Read the model definition and answer for the solid it produces. Units are mm, in the model's axes. Face numbers are marked on the shaded views. Coordinates: 2 decimals unless noted, no trailing zeros. Write each loop counter-clockwise with the first axis right and the second up, starting at its lowest first coordinate (ties: lowest second). Pieces come first, ordered by that corner, then holes. Notation, with made-up numbers: (47, -8.75) - (92, -8.75) arc R24 cw to (92, 16.25) - close; hole circle Ø2 at (-12, 47). An arc over 180 degrees is marked (long way). Use a Markdown table: item, result.
from build123d import *

# Parameters (mm, degrees)
BOSS_EXTRUDE1_DEPTH = 103
CUT_EXTRUDE2_START  = 6.04
SKETCH2_R           = 2.25
CUT_EXTRUDE2_DEPTH  = 11


with BuildPart() as part:
    # Sketch1 → Boss-Extrude1 (new body)
    with BuildSketch(Plane.XY):
        with BuildLine():
            Line((-7.5, 4.346659782), (-7.5, 0))
            ThreePointArc((-7.5, 0), (0, 2.235271482), (7.5, 0))
            Line((7.5, 0), (7.5, 4.346659782))
            ThreePointArc((7.5, 4.346659782), (0, 6.035271482), (-7.5, 4.346659782))
        make_face()
    extrude(amount=-BOSS_EXTRUDE1_DEPTH)

    # Sketch2 → Cut-Extrude2 (cut)
    with BuildSketch(Plane(origin=(0, 0, 0), x_dir=(1, 0, 0), z_dir=(0, 1, 0)).offset(CUT_EXTRUDE2_START)):
        with Locations((0, 39)):
            Circle(SKETCH2_R)
        with Locations((0, 64)):
            Circle(SKETCH2_R)
        with Locations((0, 23)):
            Circle(SKETCH2_R)
        with Locations((0, 7)):
            Circle(SKETCH2_R)
        with Locations((0, 80)):
            Circle(SKETCH2_R)
        with Locations((0, 96)):
            Circle(SKETCH2_R)
    extrude(amount=-CUT_EXTRUDE2_DEPTH, mode=Mode.SUBTRACT)

    # Sketch3 → Cut-Revolve1 (revolve, cut)
    with BuildSketch(Plane(origin=(0, 0, 0), x_dir=(0, 0, -1), z_dir=(1, 0, 0))):
        with BuildLine():
            Line((2.862670642, 6.035271482), (2.862670642, 5.235271482))
            ThreePointArc((2.862670642, 5.235271482), (3.707158189, 4.141681525), (4.75, 3.235271482))
            Line((4.75, 3.235271482), (7, 3.235271482))
            Line((7, 3.235271482), (7, 6.035271482))
            Line((7, 6.035271482), (2.862670642, 6.035271482))
        make_face()
    revolve(axis=Axis((0, 0, -7), (0, 1, 0)), mode=Mode.SUBTRACT)

    # Sketch3<3> → Cut-Revolve2 (revolve, cut)
    with BuildSketch(Plane(origin=(0, 0, 0), x_dir=(0, 0, -1), z_dir=(1, 0, 0))):
        with BuildLine():
            Line((18.862670642, 6.035271482), (18.862670642, 5.235271482))
            ThreePointArc((18.862670642, 5.235271482), (19.707158189, 4.141681525), (20.75, 3.235271482))
            Line((20.75, 3.235271482), (23, 3.235271482))
            Line((23, 3.235271482), (23, 6.035271482))
            Line((23, 6.035271482), (18.862670642, 6.035271482))
        make_face()
    revolve(axis=Axis((0, 5.890025873, -23), (0, -1, 0)), mode=Mode.SUBTRACT)

    # Sketch3<4> → Cut-Revolve3 (revolve, cut)
    with BuildSketch(Plane(origin=(0, 0, 0), x_dir=(0, 0, -1), z_dir=(1, 0, 0))):
        with BuildLine():
            Line((34.862670642, 6.035271482), (34.862670642, 5.235271482))
            ThreePointArc((34.862670642, 5.235271482), (35.707158189, 4.141681525), (36.75, 3.235271482))
            Line((36.75, 3.235271482), (39, 3.235271482))
            Line((39, 3.235271482), (39, 6.035271482))
            Line((39, 6.035271482), (34.862670642, 6.035271482))
        make_face()
    revolve(axis=Axis((0, 5.890025873, -39), (0, -1, 0)), mode=Mode.SUBTRACT)

    # Sketch3<5> → Cut-Revolve4 (revolve, cut)
    with BuildSketch(Plane(origin=(0, 0, 0), x_dir=(0, 0, -1), z_dir=(1, 0, 0))):
        with BuildLine():
            Line((59.862670642, 6.035271482), (59.862670642, 5.235271482))
            ThreePointArc((59.862670642, 5.235271482), (60.707158189, 4.141681525), (61.75, 3.235271482))
            Line((61.75, 3.235271482), (64, 3.235271482))
            Line((64, 3.235271482), (64, 6.035271482))
            Line((64, 6.035271482), (59.862670642, 6.035271482))
        make_face()
    revolve(axis=Axis((0, 5.890025873, -64), (0, -1, 0)), mode=Mode.SUBTRACT)

    # Sketch3<6> → Cut-Revolve5 (revolve, cut)
    with BuildSketch(Plane(origin=(0, 0, 0), x_dir=(0, 0, -1), z_dir=(1, 0, 0))):
        with BuildLine():
            Line((75.862670642, 6.035271482), (75.862670642, 5.235271482))
            ThreePointArc((75.862670642, 5.235271482), (76.707158189, 4.141681525), (77.75, 3.235271482))
            Line((77.75, 3.235271482), (80, 3.235271482))
            Line((80, 3.235271482), (80, 6.035271482))
            Line((80, 6.035271482), (75.862670642, 6.035271482))
        make_face()
    revolve(axis=Axis((0, 5.890025873, -80), (0, -1, 0)), mode=Mode.SUBTRACT)

    # Sketch3<7> → Cut-Revolve6 (revolve, cut)
    with BuildSketch(Plane(origin=(0, 0, 0), x_dir=(0, 0, -1), z_dir=(1, 0, 0))):
        with BuildLine():
            Line((91.862670642, 6.035271482), (91.862670642, 5.235271482))
            ThreePointArc((91.862670642, 5.235271482), (92.707158189, 4.141681525), (93.75, 3.235271482))
            Line((93.75, 3.235271482), (96, 3.235271482))
            Line((96, 3.235271482), (96, 6.035271482))
            Line((96, 6.035271482), (91.862670642, 6.035271482))
        make_face()
    revolve(axis=Axis((0, 5.890025873, -96), (0, -1, 0)), mode=Mode.SUBTRACT)


solid = part.part
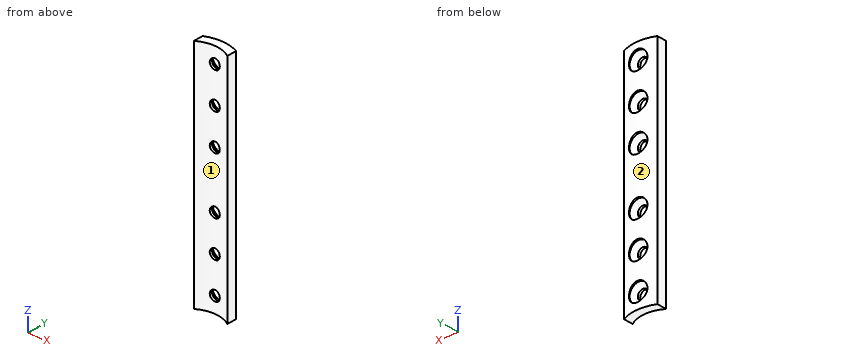
(1) A cutting plane is placed at B-B, the plane z = -91. Write down the section's boundary in (x, y).
Report:
| item | result |
|---|---|
| outline | (-7.5, 0) arc R13.7 cw to (7.5, 0) - (7.5, 4.35) arc R17.5 ccw to (-7.5, 4.35) - close |
(2) A cutting plane is placed at A-A, the plane x = 0. Count the separate pieces of the cut face and the enclosed holes in it, and give its area (3 significant figures).
Report:
| item | result |
|---|---|
| separate pieces | 7 |
| enclosed holes | 0 |
| area | 245 mm² |
(3) The mould has two halves that part along X. Classify the marked faces 1 and 2: pulls with the +X half, pulls with the -X half, needs draft (parallel to the pull), parting line crosses it, or undercut.
Report:
| item | result |
|---|---|
| face 1 | undercut |
| face 2 | parting line crosses it |
(4) Straight lines are drawn through the part: L1, parallel to X at y = 2.8, z = -23; L2, parallel to Y at x = 0, z = -54; L3, parallel to X at y = 1, z = -72.5. For each, find the intervals that lie inside material, in ascending order.
Report:
| item | result |
|---|---|
| L1 | x = -7.5 to -2.25, 2.25 to 7.5 |
| L2 | y = 2.24 to 6.04 |
| L3 | x = -7.5 to -5.69, 5.69 to 7.5 |
(5) Each of these flat-tipped pins is pushed along its axis until it touches: P1, Ø5, axis at x = 0, z = -39, coming from the -Y side; P2, Ø7, axis at x = 0, z = -23, coming from the +Y side; P3, Ø6.5, axis at x = 0, z = -96, coming from the -Y side; P4, Ø1, axis at x = 0.5, z = -47.5, coming from the +Y side. Where does it stop, or does it pass through?
Report:
| item | result |
|---|---|
| P1 | stops at y = 2.01 |
| P2 | stops at y = 4.37 |
| P3 | stops at y = 1.84 |
| P4 | stops at y = 6.04 |
(6) A cutting plane is placed at C-C, the plane x = -6. Write down the section's boundary in (y, z), and give its area (3 significant figures).
Report:
| item | result |
|---|---|
| outline | (0.85, -103) - (4.97, -103) - (4.97, 0) - (0.85, 0) - close |
| area | 425 mm² |
